Source: CAD feature listing. Evaluate the final solid. Frame: model axes, mm. A direction names the side the tool comes from. Give positions to 0.01 mm unless a question says otherwise; leave off trailing zeros. Write each loop counter-clockwise with the first axis right and the second up, starting at its lowest first coordinate (ties: lowest second). Pieces come first, ordered by that corner, then holes. Notation, with made-up numbers: (37.5, 50.5) -> (57.5, 50.5) arc R18 cw to (57.5, 74.5) -> close; hole circle Ø6 at (77, -1). An arc over 180 degrees is marked (long way). Write item = value, one per line.
from build123d import *

# Parameters (mm, degrees)
F0_W        = 25
F0_H        = 25
F0_W_2      = 21
F0_H_2      = 21
F1_DEPTH    = 200
F2_T1_DEPTH = 154.6335196453
F3_R        = 13.5
F4_DEPTH    = 25


# Not quite as in the source:
# - a fillet or chamfer that OpenCascade refuses, or shapes differently, is made with other operations: its cross-section is extruded or revolved along the edge and cut away or added


with BuildPart() as f1:
    # F0 (on Right) → F1 (new body)
    with BuildSketch(Plane.YZ):
        Rectangle(F0_W, F0_H)
        Rectangle(F0_W_2, F0_H_2, mode=Mode.SUBTRACT)
    extrude(amount=F1_DEPTH)

    # F2: chamfer of 25 x 10.3553390593 on 1 edges, made by hand

    # F2_s2 → F2_t1 (cut)
    with BuildSketch(Plane.XZ.offset(-77.3167598227)):
        Polygon((189.6446609407, 12.5), (200, -12.5), (200, 12.5), align=None)
    extrude(amount=F2_T1_DEPTH, mode=Mode.SUBTRACT)

    # F3 (on face) → F4 (cut)
    with BuildSketch(Plane.XZ.offset(12.5)):
        Circle(F3_R)
    extrude(amount=-F4_DEPTH, mode=Mode.SUBTRACT)


solid = f1.part
1) Cut plane C-C (x = 28.5). Return the cut outline in (y, z), then the cut area to 3 significant figures.
Computed:
outline = (-12.5, -12.5) -> (12.5, -12.5) -> (12.5, 12.5) -> (-12.5, 12.5) -> close; hole (-10.5, -10.5) -> (10.5, -10.5) -> (10.5, 10.5) -> (-10.5, 10.5) -> close
area = 184 mm²
2) Access query for faces 4 (the flat face through (102, 0, -10.5)), 5 (the flat face through (101, 12.5, 0)). Directions: +Z, -Z, +X, -X, +Y, -Y. A direction counts if a zero-diameter tool reaches every point of the face in a straight line with its end or side. Return the directions, or none.
Computed:
face_4 = +X, -X
face_5 = +Z, -Z, +X, -X, +Y
3) Material intervals for L1, parallel to Y at x = 77, z = -3.25; L2, parallel to Z at x = 191, y = -5, sorted ascending.
Computed:
L1 = -12.5 to -10.5, 10.5 to 12.5
L2 = -12.5 to -10.5
4) Draft query along Z for faces 1 (the flat face through (101, -12.5, 0)), 2 (the flat face through (101, 0, -12.5)), 3 (the cylindrical face through (6.5, -0.18, -11.83)). Return one class per face: pulls with the +Z half, pulls with the -Z half, needs draft (parallel to the pull), parting line crosses it, or undercut.
Computed:
face_1 = needs draft
face_2 = pulls with the -Z half
face_3 = undercut
5) Cut plane A-A (z = -1.5). Return the cut outline in (x, y), then the cut area to 3 significant figures.
Computed:
outline = (13.42, -12.5) -> (195.44, -12.5) -> (195.44, -10.5) -> (13.42, -10.5) -> close; (13.42, 10.5) -> (195.44, 10.5) -> (195.44, 12.5) -> (13.42, 12.5) -> close
area = 728 mm²
6) Cut plane B-B (y = -1). Return the cut outline in (x, z), then the cut area to 3 significant figures.
Computed:
outline = (5.1, -12.5) -> (200, -12.5) -> (199.17, -10.5) -> (8.49, -10.5) arc R13.5 cw to start; (5.1, 12.5) arc R13.5 cw to (8.49, 10.5) -> (190.47, 10.5) -> (189.64, 12.5) -> close
area = 751 mm²
